Autodesk Fusion 360 part; units mm, degrees
box "Grundkörper Quader1" add length 180 width 90 height 70 placed x (0, 0, -1) y (-1, 0, 0) z (0, 1, 0) at (19.6846, 0, 34.8152)
box "Grundkörper Quader2" cut length 179.5 width 89.5 height -10 placed x (0, 0, -1) y (-1, 0, 0) z (0, 1, 0) at (19.5, 70, 34.5)
box "Grundkörper Quader3" cut length 170 width 80 height -40 placed x (0, 0, 1) y (-1, 0, 0) z (0, -1, 0) at (15, 0, -140)
hole "Bohrung1" at (-16.4163, 60, 15.0098) direction (0, -1, 0) diameter 15 depth 40 tip angle 180
Here's how the part is built. I have some questions about the finished solid (model axes, mm). A direction names the side the tool comes from. Coordinates: 2 decimals unless noted, no trailing zeros. Write each loop counter-clockwise with the first axis right and the second up, starting at its lowest first coordinate (ties: lowest second). Pieces come first, ordered by that corner, then holes.
1) If we section it at D-D (z = -112.5): List the corners of the cut face in (x, y) for me, plus the area to 4 significant figures.
Filled in:
outline: (-70.32, 0) - (-65, 0) - (-65, 40) - (15, 40) - (15, 0) - (19.68, 0) - (19.68, 70) - (19.5, 70) - (19.5, 60) - (-70, 60) - (-70, 70) - (-70.32, 70) - close
area: 2,205 mm2
2) Which directions (+Z, -Z, +X, -X, +Y, -Y) give clear straight access to the entire face, cutting with the end or side of a thin tool? Please do faces 1 (the face through (-70, 65, -57)), 2 (the face through (15, 20, -54)), 3 (the face through (-66, 0, -55)).
Filled in:
face 1: +Y
face 2: -Y
face 3: +Z, -Z, +X, -X, -Y
3) If we section it at B-B (y = 35.5): List the corners of the cut face in (x, z) for me.
Filled in:
outline: (-70.32, -145.18) - (19.68, -145.18) - (19.68, 34.82) - (-70.32, 34.82) - close; hole (-65, -140) - (15, -140) - (15, 30) - (-65, 30) - close
4) If I drill on line 1 (X direction, y = 8.5, z = -88.5); line 2 (Z direction, x = 1, y = 29.5); line 3 (X direction, y = 67, z = -90.5), over which ranges is the centre line in solid material (lowest first)?
Filled in:
line 1: x = -70.32 to -65, 15 to 19.68
line 2: z = -145.18 to -140, 30 to 34.82
line 3: x = -70.32 to -70, 19.5 to 19.68
5) If we section it at C-C (x = -52.5): List the corners of the cut face in (y, z) for me, plus the area to 4 significant figures.
Filled in:
outline: (0, -145.18) - (70, -145.18) - (70, -145) - (60, -145) - (60, 34.5) - (70, 34.5) - (70, 34.82) - (0, 34.82) - (0, 30) - (40, 30) - (40, -140) - (0, -140) - close
area: 4,005 mm2
6) I'm going to push flat-ended pins straight in: pin 1 (5 mm diameter, centred on x = -54.5, z = -25.5, fed in from +Y); pin 2 (5 mm diameter, centred on x = -9.5, z = -5, fed in from -Y). Where does each tip first touch, or does it pass through?
Filled in:
pin 1: stops at y = 60
pin 2: stops at y = 40
7) Thinking about a two-plate mould opening in Z: for faces 4 (the face through (-26, 60, -54)), 5 (the face through (-26, 40, -56)), 6 (the face through (-25, 35, -145.185)), 7 (the face through (19.685, 35, -56)), which applies, +Z half, -Z half, draft (parallel to the pull), parting line (faces both ways), or undercut?
Filled in:
face 4: undercut
face 5: undercut
face 6: -Z half
face 7: draft
8) If we section it at A-A (z = 17.5): List the corners of the cut face in (x, y) for me, plus the area to 3 significant figures.
Filled in:
outline: (-70.32, 0) - (-65, 0) - (-65, 40) - (-23.49, 40) - (-23.49, 60) - (-70, 60) - (-70, 70) - (-70.32, 70) - close; (-9.34, 40) - (15, 40) - (15, 0) - (19.68, 0) - (19.68, 70) - (19.5, 70) - (19.5, 60) - (-9.34, 60) - close
area: 1,920 mm2
